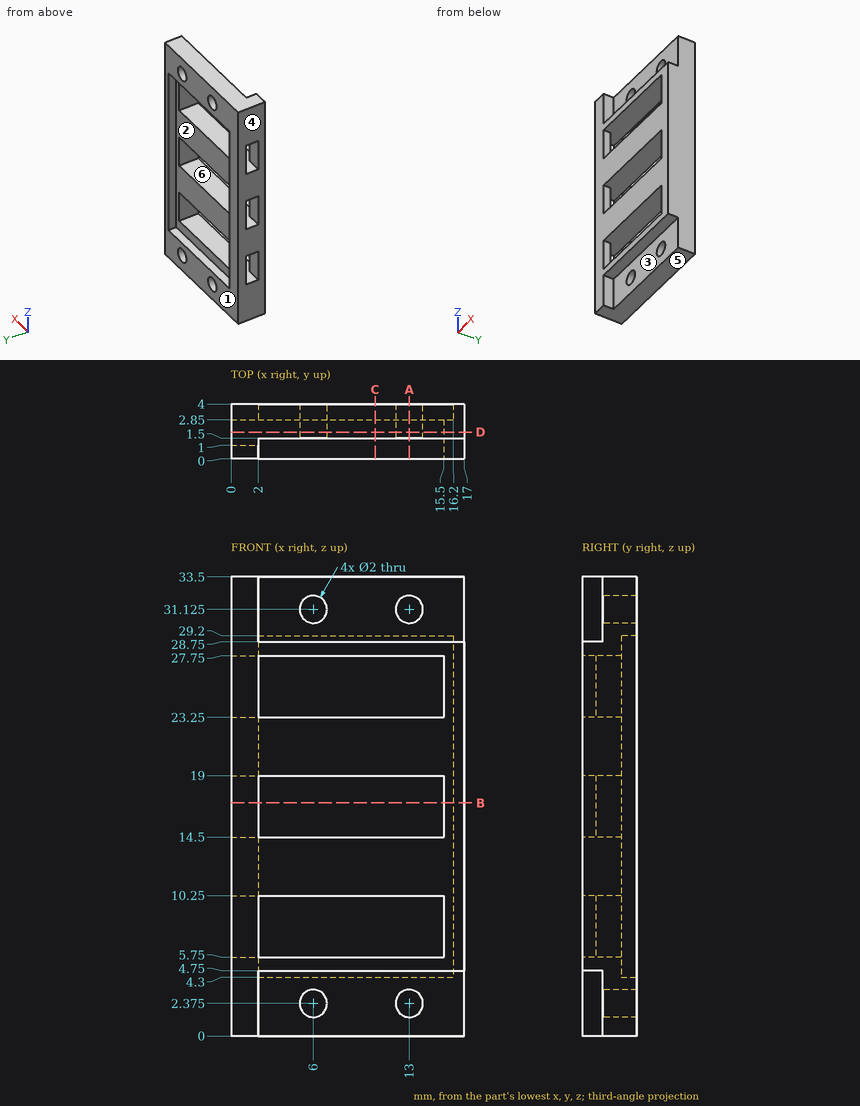
Geometry check sheet. Reference: drawing and pictorial views, mm from the part's lowest x, y, z. A direction names the side the tool comes from. Coordinates: 2 decimals unless noted, no trailing zeros. Order: outer loops, then holes, each group sorted by start corner. A loop starts at its lowest first (then second) coordinate and runs counter-clockwise, first axis right, second up. Notation, with made-up numbers: (48.5, 4) -> (97.5, 4) arc R16 ccw to (97.5, 17) -> close; hole circle Ø2 at (34.25, 36.25). An arc over 180 degrees is marked (long way). Put each result on its own line as item: value. Start each with the question number.
1) Release check for a two-part mould opening along Z. For the marked faces 4, 5 and 6 record: pulls with the +Z half, pulls with the -Z half, needs draft (parallel to the pull), parting line crosses it, or undercut.
2) Cross-section at B-B (z = 17). Enter the section's corners in (x, y).
3) Material ranges on L1, parallel to Z at x = 6, y = 3 (3 decimals); L2, parallel to Z at x = 10.25, y = 0.45; L3, parallel to Z at x = 13, y = 2.3 (3 decimals), recorded low to high.
4) Go/stop test with flat-tipped pins: pin 1 (5 mm diameter, centred on x = 13.5, z = 10, fed in from +Y); pin 2 (0.9 mm diameter, centred on y = 1.5, z = 16, fed in from -X); pin 3 (2.5 mm diameter, centred on x = 11.5, z = 1.5, fed in from -Y). Record where each tip stops, or that it passes through.
5) Cross-section at A-A (x = 13). State how many separate pieces and enclosed holes the cut face has, plus the area to 3 significant figures.
6) Tool access check on the marked faces 1, 2 and 3. Record the directions out of +Z, -Z, +X, -X, +Y, -Y that give a thin tool (end or side, any length) a straight path to the whole face; none if there is none.
7) Cross-section at D-D (y = 1.95). Enter the section's corners in (x, z) (3 decimals), plus the area to 3 significant figures.
8) Cross-section at C-C (x = 10.5). Enter the section's corners in (y, z), plus the area to 3 significant figures.
Geometry check:
1. face 4: needs draft
1. face 5: pulls with the -Z half
1. face 6: undercut
2. outline: (0, 0) -> (2, 0) -> (2, 1) -> (0, 1) -> close; (0, 2.85) -> (2, 2.85) -> (2, 4) -> (0, 4) -> close; (15.5, 0) -> (17, 0) -> (17, 4) -> (16.2, 4) -> (16.2, 2.85) -> (15.5, 2.85) -> close
3. L1: z = 0 to 1.375, 3.375 to 4.3, 29.2 to 30.125, 32.125 to 33.5
3. L2: z = 4.75 to 5.75, 10.25 to 14.5, 19 to 23.25, 27.75 to 28.75
3. L3: z = 0 to 1.375, 3.375 to 5.75, 10.25 to 14.5, 19 to 23.25, 27.75 to 30.125, 32.125 to 33.5
4. pin 1: stops at y = 2.85
4. pin 2: stops at x = 15.5
4. pin 3: stops at y = 1.5
5. separate pieces: 6
5. enclosed holes: 0
5. area: 42.6 mm^2
6. face 1: +Z, -Z, +X, -X, +Y
6. face 2: +Y
6. face 3: -Z, +X, -Y
7. outline: (0, 0) -> (17, 0) -> (17, 33.5) -> (0, 33.5) -> (0, 27.75) -> (15.5, 27.75) -> (15.5, 23.25) -> (0, 23.25) -> (0, 19) -> (15.5, 19) -> (15.5, 14.5) -> (0, 14.5) -> (0, 10.25) -> (15.5, 10.25) -> (15.5, 5.75) -> (0, 5.75) -> close; hole circle Ø2 at (6, 2.375); hole circle Ø2 at (6, 31.125); hole circle Ø2 at (13, 2.375); hole circle Ø2 at (13, 31.125)
7. area: 348 mm^2
8. outline: (0, 4.75) -> (1.5, 4.75) -> (1.5, 0) -> (4, 0) -> (4, 4.3) -> (2.85, 4.3) -> (2.85, 5.75) -> (0, 5.75) -> close; (0, 10.25) -> (2.85, 10.25) -> (2.85, 14.5) -> (0, 14.5) -> close; (0, 19) -> (2.85, 19) -> (2.85, 23.25) -> (0, 23.25) -> close; (0, 27.75) -> (2.85, 27.75) -> (2.85, 29.2) -> (4, 29.2) -> (4, 33.5) -> (1.5, 33.5) -> (1.5, 28.75) -> (0, 28.75) -> close
8. area: 52.6 mm^2
